```python
from build123d import *

# Parameters (mm, degrees)
ESTRUSIONE_ESTRUSIONE1_DEPTH  = 27
TAGLIO_ESTRUSIONE1_DEPTH      = 27
TAGLIO_ESTRUSIONE1_DEPTH_BACK = 27
SCHIZZO2_W                    = 4
SCHIZZO2_H                    = 8.25
SCHIZZO2_R                    = 2


with BuildPart() as part:
    # Schizzo1 → Estrusione-Estrusione1 (new body)
    with BuildSketch(Plane.XY):
        with BuildLine():
            Line((-8, 1), (8, 1))
            ThreePointArc((8, 1), (9.299038106, 3.25), (6.700961894, 3.25))
            Line((6.700961894, 3.25), (5.834936491, 3.75))
            ThreePointArc((5.834936491, 3.75), (10.165063509, 3.75), (8, 0))
            Line((8, 0), (-8, 0))
            Line((-8, 0), (-8, 1))
        make_face()
    extrude(amount=ESTRUSIONE_ESTRUSIONE1_DEPTH)

    # Schizzo2 → Taglio-Estrusione1 (cut, two sides: drawn at the far end of the back side and taken through both)
    with BuildSketch(Plane(origin=(0, 1, 0), x_dir=(1, 0, 0), z_dir=(0, 1, 0)).offset(-TAGLIO_ESTRUSIONE1_DEPTH_BACK)):
        with BuildLine():
            Line((8, -27), (8, -18.75))
            Line((8, -18.75), (2.509224592, -18.75))
            ThreePointArc((2.509224592, -18.75), (2.055446947, -18.858885053), (1.700488507, -19.161828302))
            Line((1.700488507, -19.161828302), (-2.166002653, -24.478253647))
            ThreePointArc((-2.166002653, -24.478253647), (-3.967228406, -25.293451017), (-5.588882762, -24.162434609))
            ThreePointArc((-5.588882762, -24.162434609), (-7.389705753, -18.965825604), (-8, -13.5))
            Line((-8, -13.5), (-8, -27))
            Line((-8, -27), (8, -27))
        make_face()
        with BuildLine():
            Line((2.509224592, -8.25), (8, -8.25))
            Line((8, -8.25), (8, 0))
            Line((8, 0), (-8, 0))
            Line((-8, 0), (-8, -13.5))
            ThreePointArc((-8, -13.5), (-7.389705753, -8.034174396), (-5.588882762, -2.837565391))
            ThreePointArc((-5.588882762, -2.837565391), (-3.967228406, -1.706548983), (-2.166002653, -2.521746353))
            Line((-2.166002653, -2.521746353), (1.700488507, -7.838171698))
            ThreePointArc((1.700488507, -7.838171698), (2.055446947, -8.141114947), (2.509224592, -8.25))
        make_face()
        with Locations((10, -22.875)):
            Rectangle(SCHIZZO2_W, SCHIZZO2_H)
        with Locations((10, -4.125)):
            Rectangle(SCHIZZO2_W, SCHIZZO2_H)
        with Locations((-4, -20)):
            Circle(SCHIZZO2_R)
        with Locations((-4, -7)):
            Circle(SCHIZZO2_R)
    extrude(amount=TAGLIO_ESTRUSIONE1_DEPTH + TAGLIO_ESTRUSIONE1_DEPTH_BACK, mode=Mode.SUBTRACT)


solid = part.part
```
CAD build for the part. Positions are in the model's coordinates, mm. A direction names the side the tool comes from. Round coordinates to 2 decimals unless told otherwise and drop trailing zeros. Order: outer loops, then holes, each group sorted by start corner. A loop starts at its lowest first (then second) coordinate and runs counter-clockwise, first axis right, second up.
Q1. Slice it at B-B (x = 6.25). Write the cut outline in (y, z).
Q2. Two-plate mould, pull along X, no slides. Class faces 4 (the cylindrical face through (-4.26, 0.493, 18.017)), 5 (the cylindrical face through (2.05, 0.49, 8.14)), 6 (the flat face through (7.4, 0.8, 18.75)): pulls with the +X half, pulls with the -X half, needs draft (parallel to the pull), parting line crosses it, or undercut.
Q3. Wall check: L1, parallel to Z at x = -4, y = 0.65; L2, parallel to Z at x = -4.25, y = 0.6; L3, parallel to Y at x = -3.75, z = 10.5. Give the ranges that are in metal, low to high.
Q4. Slice it at C-C (x = -4). Write the cut outline in (y, z), and give its area (3 significant figures).
Q5. Slice it at A-A (z = 5.5). Write the cut outline in (x, y).
Q6. Slice it at D-D (y = 2). Write the cut outline in (x, z).
Q7. Drop flat-ended pins along their axis: pin 1 (8 mm diameter, centred on x = -2.5, z = 12, fed in from +Y); pin 2 (2.5 mm diameter, centred on x = 7.5, y = 3.5, fed in from +Z); pin 3 (2 mm diameter, centred on x = 6.5, y = 1.5, fed in from -Z). Give the stop position or say it passes through.
Q8. Which spindle directions (+Z, -Z, +X, -X, +Y, -Y) get a long thin tool onto all of the face, cutting with end or side? Do faces 1 (the cylindrical face through (9.32, 3.21, 13.43)), 2 (the flat face through (6.27, 3.5, 13.43)), 3 (the flat face through (7.3, 0.8, 8.25)). Say none if no direction does.
Results below:
1. outline: (0, 8.25) - (1, 8.25) - (1, 18.75) - (0, 18.75) - close; (3.51, 8.25) - (4.29, 8.25) - (4.29, 18.75) - (3.51, 18.75) - close
2. face 4: undercut
2. face 5: pulls with the +X half
2. face 6: needs draft
3. L1: z = 1.71 to 5, 9 to 18, 22 to 25.29
3. L2: z = 1.75 to 5.02, 8.98 to 18.02, 21.98 to 25.25
3. L3: y = 0 to 1
4. outline: (0, 1.71) - (1, 1.71) - (1, 5) - (0, 5) - close; (0, 9) - (1, 9) - (1, 18) - (0, 18) - close; (0, 22) - (1, 22) - (1, 25.29) - (0, 25.29) - close
4. area: 15.6 mm2
5. outline: (-6.67, 0) - (-5.32, 0) - (-5.32, 1) - (-6.67, 1) - close; (-2.68, 0) - (0, 0) - (0, 1) - (-2.68, 1) - close
6. outline: (9.41, 8.25) - (10.45, 8.25) - (10.45, 18.75) - (9.41, 18.75) - close
7. pin 1: stops at y = 1
7. pin 2: stops at z = 18.75
7. pin 3: stops at z = 8.25
8. face 1: +Z, -Z
8. face 2: +Z, -Z, -X
8. face 3: -Z, +X, +Y, -Y
